```python
from build123d import *

# Parameters (mm, degrees)
F_3_8_NPT_TAPPED_HOLE1_AT_2_COUNT = 2
F_3_8_NPT_TAPPED_HOLE1_AT_2_PITCH = 76.2
F_3_8_CLEARANCE_HOLE2_D           = 10.0838
CIRPATTERN1_COUNT                 = 10
SKETCH15_R                        = 3.175
CUT_EXTRUDE1_DEPTH                = 12.7


with BuildPart() as part:
    # Sketch1 → Revolve1 (revolve)
    with BuildSketch(Plane.XY):
        Polygon((0, 0), (-76.2, 0), (-76.2, -38.1), (-60.96, -38.1), (-60.96, -32.258), (-55.7149, -32.258), (-55.7149, -29.5656), (-51.6509, -29.5656), (-51.6509, -32.258), (-32.163982831, -32.258), (-30.364664072, -32.258), (-28.575, -32.258), (-28.575, -27.178), (-28.0924, -27.178), (-28.0924, -24.4856), (-24.0284, -24.4856), (-24.0284, -27.178), (-22.225, -27.178), (0, -15.85722), align=None)
    revolve(axis=Axis((0, 0, 0), (0, -1, 0)))

    # Sketch3 → 1/2 NPT Tapped Hole1 (revolve, cut)
    with BuildSketch(Plane(origin=(0, 0, 0), x_dir=(0, 0, 1), z_dir=(1, 0, 0))):
        Polygon((0, 0), (0, 38.1), (8.9281, 38.1), (8.9281, 13.462), (10.261665792, 13.462), (10.6647361, 0), align=None)
    revolve(axis=Axis((0, 6.35, 0), (0, -1, 0)), mode=Mode.SUBTRACT)

    # Sketch5 → 3/8 NPT Tapped Hole1 (revolve, cut)
    with BuildSketch(Plane(origin=(-38.1, 0, 0), x_dir=(0, 0, 1), z_dir=(1, 0, 0))):
        Polygon((0, 0), (0, 38.1), (7.1374, 38.1), (7.1374, 10.414), (8.263205494, 10.414), (8.5750146, 0), align=None)
    f_3_8_npt_tapped_hole1 = revolve(axis=Axis((-38.1, 6.35, 0), (0, -1, 0)), mode=Mode.SUBTRACT)

    # 3/8 NPT Tapped Hole1 at 2: 3/8 NPT Tapped Hole1 ×2
    with Locations(*[(i * F_3_8_NPT_TAPPED_HOLE1_AT_2_PITCH, 0, 0) for i in range(1, F_3_8_NPT_TAPPED_HOLE1_AT_2_COUNT)]):
        add(f_3_8_npt_tapped_hole1, mode=Mode.SUBTRACT)

    # 3/8 Clearance Hole2 (through all)
    with Locations(Plane(origin=(67.31, 0, 0), x_dir=(1, 0, 0), z_dir=(0, 1, 0))):
        with Locations((0, 0)):
            f_3_8_clearance_hole2 = Hole(F_3_8_CLEARANCE_HOLE2_D / 2)

    # CirPattern1: 3/8 Clearance Hole2 ×10 about axis
    cirpattern1_axis = Axis((0, 0, 0), (0, 1, 0))
    for i in range(1, CIRPATTERN1_COUNT):
        add(f_3_8_clearance_hole2.rotate(cirpattern1_axis, i * 360 / CIRPATTERN1_COUNT), mode=Mode.SUBTRACT)

    # Sketch7 → 1/8 NPT Tapped Hole2 (revolve, cut)
    with BuildSketch(Plane(origin=(19.05, 0, -33.02), x_dir=(0, 0, 1), z_dir=(1, 0, 0))):
        Polygon((0, 0), (0, 38.1), (4.2164, 38.1), (4.2164, 6.858), (4.556413846, 6.858), (4.7427388, 0.635), (5.3777388, 0), align=None)
    revolve(axis=Axis((19.05, 6.35, -33.02), (0, -1, 0)), mode=Mode.SUBTRACT)

    # Sketch15 → Cut-Extrude1 (cut, symmetric)
    with BuildSketch(Plane(origin=(0, -4.272551224, -4.272551224), x_dir=(0, 0.7071067811865489, -0.7071067811865461), z_dir=(0, -0.7071067811865461, -0.7071067811865489))):
        with Locations((-30.172299887, 0)):
            Circle(SKETCH15_R)
    extrude(amount=CUT_EXTRUDE1_DEPTH, both=True, mode=Mode.SUBTRACT)

    # Sketch12 → 1/8 NPT Tapped Hole3 (revolve, cut)
    with BuildSketch(Plane(origin=(0, 0, 26.67), x_dir=(0, 0, 1), z_dir=(1, 0, 0))):
        Polygon((0, 0), (0, 20.32), (4.2164, 17.786531286), (4.2164, 6.858), (4.543696598, 6.858), (4.7427388, 0.2102612), (4.953, 0), align=None)
    revolve(axis=Axis((0, 6.35, 26.67), (0, -1, 0)), mode=Mode.SUBTRACT)

    # Sketch17 → 1/4 NPT Tapped Hole1 (revolve, cut)
    with BuildSketch(Plane(origin=(-19.05, 0, -33.02), x_dir=(0, 0, 1), z_dir=(1, 0, 0))):
        Polygon((0, 0), (0, 38.1), (5.5626, 38.1), (5.5626, 9.906), (5.962698545, 9.906), (6.2402847, 0.635), (6.8752847, 0), align=None)
    revolve(axis=Axis((-19.05, 6.35, -33.02), (0, -1, 0)), mode=Mode.SUBTRACT)


solid = part.part
```
Can you work these out from the model? Positions are in its coordinate system, mm. A direction names the side the tool comes from. Coordinates: 2 decimals unless noted, no trailing zeros. Order: outer loops, then holes, each group sorted by start corner. A loop starts at its lowest first (then second) coordinate and runs counter-clockwise, first axis right, second up. Notation, with made-up numbers: (2.25, 43) -> (46.25, 43) arc R20 ccw to (46.25, 81) -> close; hole circle Ø1 at (77.5, 71.25). An arc over 180 degrees is marked (long way). Write each question's results on one line, items separated by ' | '.
Item 1: If I drill on line 1 along X through (y, z) = (-26, 38); line 2 along Z through (x, y) = (-1, -8); line 3 along X through (y, z) = (-14, 35.5), over which ranges is the centre line in solid material (lowest first)?
Results are:
line 1: -66.05 to -59.25, -49.66 to 49.66, 59.25 to 66.05 | line 2: -76.19 to -10.38, 10.38 to 22.57, 30.77 to 76.19 | line 3: -67.43 to -57.44, -51.47 to 51.47, 57.44 to 67.43
Item 2: I'm going to push flat-ended pins straight in: pin 1 Ø1 at (y, z) = (-29.5, -3.5) entering from +X; pin 2 Ø6 at (x, y) = (0.5, -20) entering from +Z; pin 3 Ø8 at (x, y) = (-19, -6) entering from +Z. Where does each tip first touch, or does it pass through?
Results are:
pin 1: x = 76.14 | pin 2: z = 76.2 | pin 3: z = 74.71
Item 3: I want a section at A-A, the plane z = 40.5. Write out the boundary of the cut face in (x, y), then the cut area to 3 significant figures.
Results are:
outline: (-64.55, -38.1) -> (-59.41, -38.1) -> (-59.41, 0) -> (-64.55, 0) -> close; (-49.5, -38.1) -> (-45.56, -38.1) -> (-45.56, -32.26) -> (-38.26, -32.26) -> (-38.26, -29.57) -> (-32.06, -29.57) -> (-32.06, -32.26) -> (32.06, -32.26) -> (32.06, -29.57) -> (38.26, -29.57) -> (38.26, -32.26) -> (45.56, -32.26) -> (45.56, -38.1) -> (49.5, -38.1) -> (49.5, 0) -> (-49.5, 0) -> close; (59.41, -38.1) -> (64.55, -38.1) -> (64.55, 0) -> (59.41, 0) -> close | area: 3,600 mm²
Item 4: I want a section at B-B, the plane y = -5. Count the separate pieces of the cut face and the enclosed holes in it, then the cut area to 3 significant figures.
Results are:
separate pieces: 1 | enclosed holes: 16 | area: 16,400 mm²
Item 5: Which directions (+Z, -Z, +X, -X, +Y, -Y) give clear straight access to the entire face, cutting with the end or side of a thin tool? Please do faces 1 (the face through (-36, -10.414, 7)), 2 (the face through (-21, -27.178, 19)), 3 (the face through (17.78, -19.38, -29)).
Results are:
face 1: +Y | face 2: -Y | face 3: +Y, -Y
Item 6: If we mould it in two halves opening along Z, with no side actions, what happens to faces 4 (the face through (28.547, -29.682, -1.256)), 5 (the face through (16, 0, -1))? For each: +Z half, -Z half, draft (parallel to the pull), parting line (faces both ways), or undercut.
Results are:
face 4: undercut | face 5: draft
Item 7: I want a section at D-D, the plane x = -67.31. Write out the boundary of the cut face in (y, z), then the cut area to 3 significant figures.
Results are:
outline: (-38.1, -35.72) -> (0, -35.72) -> (0, -5.04) -> (-38.1, -5.04) -> close; (-38.1, 5.04) -> (0, 5.04) -> (0, 35.72) -> (-38.1, 35.72) -> close | area: 2,340 mm²
Item 8: I want a section at C-C, the plane x = -38.1. Write out the boundary of the cut face in (y, z).
Results are:
outline: (-38.1, -65.99) -> (0, -65.99) -> (0, -8.58) -> (-10.41, -8.26) -> (-10.41, -7.14) -> (-32.26, -7.14) -> (-32.26, -34.87) -> (-29.57, -34.87) -> (-29.57, -40.65) -> (-32.26, -40.65) -> (-32.26, -47.59) -> (-38.1, -47.59) -> close; (-38.1, 47.59) -> (-32.26, 47.59) -> (-32.26, 40.65) -> (-29.57, 40.65) -> (-29.57, 34.87) -> (-32.26, 34.87) -> (-32.26, 7.14) -> (-10.41, 7.14) -> (-10.41, 8.26) -> (0, 8.58) -> (0, 65.99) -> (-38.1, 65.99) -> close
